Check sheet for the modelled part. Datum: model origin and axes. Units: mm. Face numbers are marked on the shaded views. A direction names the side the tool comes from. Round coordinates to 2 decimals unless told otherwise and drop trailing zeros. Order: outer loops, then holes, each group sorted by start corner. A loop starts at its lowest first (then second) coordinate and runs counter-clockwise, first axis right, second up. Notation, with made-up numbers: (26, 79) -> (47, 79) arc R7 cw to (47, 84) -> close; hole circle Ø6 at (-8.5, -25.75). An arc over 180 degrees is marked (long way). Answer in a Markdown table with one row per item.
```python
from build123d import *
from build123d.topology import SkipClean

# Parameters (mm, degrees)
SKETCH3_R             = 1.75
STIR_BAR_DEPTH        = 10
SKETCH4_W             = 10.5
SKETCH4_H             = 0.25
STIR_BAR_HOLDER_ANGLE = 180
BOSS_EXTRUDE1_DEPTH   = 2.25
SKETCH10_R            = 5.711829829
SKETCH10_R_2          = 5
CUT_EXTRUDE5_DEPTH    = 12.624328088
SKETCH9_R             = 1.75
CUT_EXTRUDE6_DEPTH    = 12.404494879


with BuildPart() as part:
    # Sketch3 → Stir Bar (new body)
    with BuildSketch(Plane(origin=(0, 0, 0), x_dir=(0, 0, -1), z_dir=(1, 0, 0))):
        Circle(SKETCH3_R)
    extrude(amount=STIR_BAR_DEPTH)



with BuildPart() as body_2:
    # Sketch4 → Stir Bar Holder (revolve)
    with BuildSketch(Plane(origin=(0, 0, 0), x_dir=(1, 0, 0), z_dir=(0, 1, 0))):
        with Locations((5, 2.125)):
            Rectangle(SKETCH4_W, SKETCH4_H)
    revolve(axis=Axis((-0.25, 0, 0), (1, 0, 0)), revolution_arc=STIR_BAR_HOLDER_ANGLE)


with BuildPart() as part_1:
    with SkipClean():  # the faces are left unmerged after this step: merging them gives an invalid solid
        add(part.part)

        add(body_2.part)  # Boss-Extrude1 merges body 2
        # Sketch5 → Boss-Extrude1 (add, through all)
        with BuildSketch(Plane.XZ):
            with BuildLine():
                ThreePointArc((0.987831011, 2.25), (5, 4.6), (9.012168989, 2.25))
                Line((9.012168989, 2.25), (9.465142775, 2.25))
                ThreePointArc((9.465142775, 2.25), (5, 5), (0.534857225, 2.25))
                Line((0.534857225, 2.25), (0.987831011, 2.25))
            make_face()
            with BuildLine():
                ThreePointArc((9.012168989, 2.25), (9.079231651, 2.125998385), (9.142463035, 2))
                Line((9.142463035, 2), (9.582575695, 2))
                ThreePointArc((9.582575695, 2), (9.52558586, 2.125811051), (9.465142775, 2.25))
                Line((9.465142775, 2.25), (9.012168989, 2.25))
            make_face()
            with BuildLine():
                Line((0.417424305, 2), (0.857536965, 2))
                ThreePointArc((0.857536965, 2), (0.920768349, 2.125998385), (0.987831011, 2.25))
                Line((0.987831011, 2.25), (0.534857225, 2.25))
                ThreePointArc((0.534857225, 2.25), (0.47441414, 2.125811051), (0.417424305, 2))
            make_face()
            with BuildLine():
                ThreePointArc((9.142463035, 2), (9.484157109, 1.025833816), (9.6, 0))
                Line((9.6, 0), (10, 0))
                ThreePointArc((10, 0), (9.894531565, 1.021548218), (9.582575695, 2))
                Line((9.582575695, 2), (9.142463035, 2))
            make_face()
            with BuildLine():
                Line((0, 0), (0.4, 0))
                ThreePointArc((0.4, 0), (0.515842891, 1.025833816), (0.857536965, 2))
                Line((0.857536965, 2), (0.417424305, 2))
                ThreePointArc((0.417424305, 2), (0.105468435, 1.021548218), (0, 0))
            make_face()
            with BuildLine():
                Line((10, 0), (9.6, 0))
                ThreePointArc((9.6, 0), (5, -4.6), (0.4, 0))
                Line((0.4, 0), (0, 0))
                ThreePointArc((0, 0), (5, -5), (10, 0))
            make_face()
        extrude(amount=-BOSS_EXTRUDE1_DEPTH)

    # Sketch10 → Cut-Extrude5 (cut, through all)
    with BuildSketch(Plane.XZ):
        with Locations((5, 0)):
            Circle(SKETCH10_R)
        with Locations(Location((5, 0, 0), (0, 0, 270))):
            Circle(SKETCH10_R_2, mode=Mode.SUBTRACT)
    extrude(amount=-CUT_EXTRUDE5_DEPTH, mode=Mode.SUBTRACT)

    # Sketch9 → Cut-Extrude6 (cut, through all)
    with BuildSketch(Plane.ZY):
        Circle(SKETCH9_R)
    extrude(amount=-CUT_EXTRUDE6_DEPTH, mode=Mode.SUBTRACT)


solid = part_1.part
```
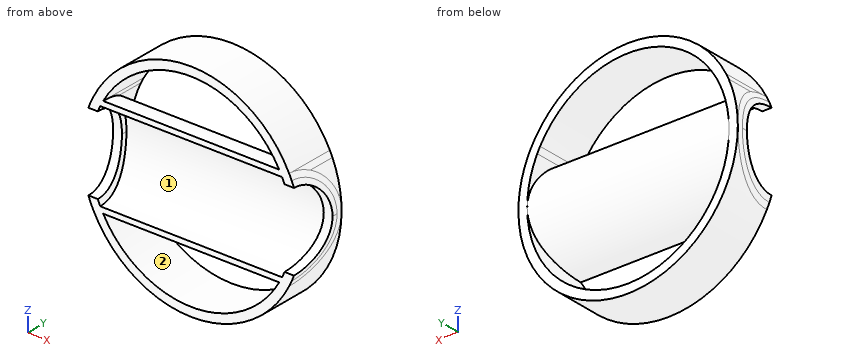
(1) Section check B-B on y = 1.4. Record the boundary of the cut face in (x, z), plus the area to 3 significant figures.
Solutions:
| item | result |
|---|---|
| outline | (0.11, -1.05) arc R5 ccw to (9.89, -1.05) -> (9.48, -1.05) arc R4.6 cw to (9.37, -1.43) -> (0.63, -1.43) arc R4.6 cw to (0.52, -1.05) -> close; (0.11, 1.05) -> (0.52, 1.05) arc R4.6 cw to (0.63, 1.43) -> (9.37, 1.43) arc R4.6 cw to (9.48, 1.05) -> (9.89, 1.05) arc R5 ccw to start; hole (0.75, -1.76) arc R4.6 ccw to (9.25, -1.76) -> close; hole (0.75, 1.76) -> (9.25, 1.76) arc R4.6 ccw to start |
| area | 16.1 mm^2 |
(2) Section check D-D on x = 2. Record the boundary of the cut face in (y, z), plus the area to 3 significant figures.
Solutions:
| item | result |
|---|---|
| outline | (0, -4) -> (2.25, -4) -> (2.25, -3.49) -> (0, -3.49) -> close; (0, -2.25) arc R2.25 ccw to (0, 2.25) -> (0, 2) arc R2 cw to (0, -2) -> close; (0, 3.49) -> (2.25, 3.49) -> (2.25, 4) -> (0, 4) -> close |
| area | 3.98 mm^2 |
(3) Tool access check on the marked faces 1 and 2. Record the directions out of +Z, -Z, +X, -X, +Y, -Y that give a thin tool (end or side, any length) a straight path to the whole face; none if there is none.
Solutions:
| item | result |
|---|---|
| face 1 | -Y |
| face 2 | +Y |
(4) Scan lines: probe 1 along Z at (x, y) = (9, 1.65); probe 2 along Z at (x, y) = (8.5, 0.85); probe 3 along X at (y, z) = (1.6, -3.25). Record each from-to range of solid material in increasing order. Write a range as from..to.
Solutions:
| item | result |
|---|---|
| probe 1 | -3..-2.27, -1.53..-1.13, 1.13..1.53, 2.27..3 |
| probe 2 | -3.57..-2.98, -2.08..-1.81, 1.81..2.08, 2.98..3.57 |
| probe 3 | 1.2..1.74, 8.26..8.8 |
(5) Section check A-A on x = 5. Record the boundary of the cut face in (y, z).
Solutions:
| item | result |
|---|---|
| outline | (0, -5) -> (2.25, -5) -> (2.25, -4.6) -> (0, -4.6) -> close; (0, -2.25) arc R2.25 ccw to (0, 2.25) -> (0, 2) arc R2 cw to (0, -2) -> close; (0, 4.6) -> (2.25, 4.6) -> (2.25, 5) -> (0, 5) -> close |
(6) Section check C-C on z = -3. Record the boundary of the cut face in (x, y), plus the area to 3 significant figures.
Solutions:
| item | result |
|---|---|
| outline | (1, 0) -> (1.51, 0) -> (1.51, 2.25) -> (1, 2.25) -> close; (8.49, 0) -> (9, 0) -> (9, 2.25) -> (8.49, 2.25) -> close |
| area | 2.31 mm^2 |
